Here's how the part is built. I have some questions about the finished solid (model axes, mm). A direction names the side the tool comes from. Coordinates: 2 decimals unless noted, no trailing zeros. Write each loop counter-clockwise with the first axis right and the second up, starting at its lowest first coordinate (ties: lowest second). Pieces come first, ordered by that corner, then holes. Notation, with made-up numbers: M 59.25,27 L 99.25,27 A30 cw 99.25,54 Z; hole C 7,75.25 d2. An arc over 180 degrees is marked long. Write each question's results on one line, items separated by ' | '. Start each with the question number.
from build123d import *

# Parameters (mm, degrees)
F1_DEPTH = 4.4958
F3_DEPTH = 3.175
F5_DEPTH = 3.175
F7_DEPTH = 2.54
F9_DEPTH = 24.004


with BuildPart() as f1:
    # F0 (on Top) → F1 (new body)
    with BuildSketch(Plane.XY):
        with BuildLine():
            Line((-10.254373, 5.965228), (-10.254373, -0.308572))
            Line((-10.254373, -0.308572), (-10.254373, -9.70656))
            Line((-10.254373, -9.70656), (-8.895473, -18.088572))
            Line((-8.895473, -18.088572), (9.214727, -18.088572))
            Line((9.214727, -18.088572), (10.573627, -9.70656))
            Line((10.573627, -9.70656), (10.573627, -0.308572))
            Line((10.573627, -0.308572), (10.573627, 5.965228))
            Line((10.573627, 5.965228), (10.573627, 6.803428))
            Line((10.573627, 6.803428), (8.071727, 6.803428))
            Line((8.071727, 6.803428), (8.071727, -1.197572))
            ThreePointArc((8.071727, -1.197572), (7.789027, -1.880072), (7.106527, -2.162772))
            ThreePointArc((7.106527, -2.162772), (6.424028, -1.880072), (6.141327, -1.197572))
            Line((6.141327, -1.197572), (6.141327, 6.803428))
            Line((6.141327, 6.803428), (-5.974473, 6.803428))
            Line((-5.974473, 6.803428), (-5.974473, -1.197572))
            ThreePointArc((-5.974473, -1.197572), (-6.257173, -1.880072), (-6.939673, -2.162772))
            ThreePointArc((-6.939673, -2.162772), (-7.622172, -1.880072), (-7.904873, -1.197572))
            Line((-7.904873, -1.197572), (-7.904873, 6.803428))
            Line((-7.904873, 6.803428), (-10.254373, 6.803428))
            Line((-10.254373, 6.803428), (-10.254373, 5.965228))
        make_face()
    extrude(amount=F1_DEPTH)

    # F2 (on face) → F3 (join)
    with BuildSketch(Plane.YZ.offset(10.573627)):
        with BuildLine():
            Line((4.555528, 2.2479), (4.555528, 4.2799))
            ThreePointArc((4.555528, 4.2799), (2.523528, 2.2479), (4.555528, 0.2159))
            Line((4.555528, 0.2159), (4.555528, 2.2479))
        make_face()
        with BuildLine():
            ThreePointArc((4.555528, 0.2159), (5.992369, 0.811059), (6.587528, 2.2479))
            ThreePointArc((6.587528, 2.2479), (5.992369, 3.684741), (4.555528, 4.2799))
            Line((4.555528, 4.2799), (4.555528, 2.2479))
            Line((4.555528, 2.2479), (4.555528, 0.2159))
        make_face()
    extrude(amount=F3_DEPTH)

    # F4 (on face) → F5 (join)
    with BuildSketch(Plane(origin=(-10.254373, 0, 0), x_dir=(0, -1, 0), z_dir=(-1, 0, 0))):
        with BuildLine():
            Line((-4.555528, 2.2479), (-4.555528, 4.2799))
            ThreePointArc((-4.555528, 4.2799), (-5.992369, 3.684741), (-6.587528, 2.2479))
            ThreePointArc((-6.587528, 2.2479), (-5.992369, 0.811059), (-4.555528, 0.2159))
            Line((-4.555528, 0.2159), (-4.555528, 2.2479))
        make_face()
        with BuildLine():
            ThreePointArc((-4.555528, 0.2159), (-3.118687, 0.811059), (-2.523528, 2.2479))
            ThreePointArc((-2.523528, 2.2479), (-3.118687, 3.684741), (-4.555528, 4.2799))
            Line((-4.555528, 4.2799), (-4.555528, 2.2479))
            Line((-4.555528, 2.2479), (-4.555528, 0.2159))
        make_face()
    extrude(amount=F5_DEPTH)

    # F6 (on face) → F7 (cut)
    with BuildSketch(Plane.XY.offset(4.4958)):
        with BuildLine():
            ThreePointArc((-5.974473, -1.197572), (-6.939673, -2.162772), (-7.904873, -1.197572))
            Line((-7.904873, -1.197572), (-7.904873, -9.70656))
            Line((-7.904873, -9.70656), (-6.545973, -18.088572))
            Line((-6.545973, -18.088572), (6.712827, -18.088572))
            Line((6.712827, -18.088572), (8.071727, -9.70656))
            Line((8.071727, -9.70656), (8.071727, -1.197572))
            ThreePointArc((8.071727, -1.197572), (7.106527, -2.162772), (6.141327, -1.197572))
            Line((6.141327, -1.197572), (6.141327, 6.803428))
            Line((6.141327, 6.803428), (-5.974473, 6.803428))
            Line((-5.974473, 6.803428), (-5.974473, -1.197572))
        make_face()
    extrude(amount=-F7_DEPTH, mode=Mode.SUBTRACT)

    # F8 (on face) → F9 (cut, through all)
    with BuildSketch(Plane.YZ.offset(10.573627)):
        Polygon((-18.088572, 4.4958), (-18.088572, 0), (-16.818572, 4.4958), align=None)
    extrude(amount=-F9_DEPTH, mode=Mode.SUBTRACT)


solid = f1.part
1) I want a section at D-D, the plane x = 8.5. Write out the boundary of the cut face in (y, z).
2) We'd pull the mould along X, two halves only. Please class faces 4 (the flat face through (10.574, -3, 2)), 5 (the flat face through (-7.905, 0, 3)), 6 (the flat face through (-9, 6.803, 2)): pulls with the +X half, pulls with the -X half, needs draft (parallel to the pull), parting line crosses it, or undercut.
3) I want a section at C-C, the plane y = -8.25. Write out the boundary of the cut face in (x, z).
4) I want a section at B-B, the plane z = 2.75. Write out the boundary of the cut face in (x, y), then the cut area to 3 significant figures.
5) For pin 1 Ø1.3 at (y, z) = (-3.5, 1) entering from -X; pin 2 Ø2 at (x, y) = (-3, -14.5) entering from +Z; pin 3 Ø2 at (y, z) = (-13.5, 2) entering from +X, each with a flat end and sliding along its axis, tell me the tip position at first contact or that it passes through.
6) For faces 1 (the flat face through (0, -5, 1.956)), 2 (the flat face through (9, 6.803, 2)), 3 (the flat face through (-5.974, 3, 1)), which set-ups out of +Z, -Z, +X, -X, +Y, -Y let a thin tool reach every point of the face, with its end or its side?
7) I want a section at A-A, the plane y = 1.5. Write out the boundary of the cut face in (x, z).
8) Please list where these lines run through material, in increasing order: line 1 (X direction, y = 2, z = 1.1); line 2 (X direction, y = 1.25, z = 3.25); line 3 (Z direction, x = -1.25, y = 0). Write a range as [from, to].
Output:
1) outline: M -18.09,0 L 6.8,0 L 6.8,4.5 L -16.82,4.5 Z
2) face 4: pulls with the +X half | face 5: undercut | face 6: needs draft
3) outline: M -10.25,0 L 10.57,0 L 10.57,4.5 L 8.07,4.5 L 8.07,1.96 L -7.9,1.96 L -7.9,4.5 L -10.25,4.5 Z
4) outline: M -13.43,2.59 L -10.25,2.59 L -10.25,-9.71 L -9.02,-17.31 L -6.67,-17.31 L -7.9,-9.71 L -7.9,6.8 L -10.25,6.8 L -10.25,6.52 L -13.43,6.52 Z; M 6.84,-17.31 L 9.34,-17.31 L 10.57,-9.71 L 10.57,2.59 L 13.75,2.59 L 13.75,6.52 L 10.57,6.52 L 10.57,6.8 L 8.07,6.8 L 8.07,-9.71 Z | area: 142 mm2
5) pin 1: stops at x = -10.25 | pin 2: stops at z = 1.96 | pin 3: stops at x = 10.12
6) face 1: +Z, +Y | face 2: +Z, -Z, +X, -X, +Y | face 3: +Z, -Z, +Y
7) outline: M -10.25,0 L -7.9,0 L -7.9,4.5 L -10.25,4.5 Z; M -5.97,0 L 6.14,0 L 6.14,1.96 L -5.97,1.96 Z; M 8.07,0 L 10.57,0 L 10.57,4.5 L 8.07,4.5 Z
8) line 1: x = [-10.25, -7.9], [-5.97, 6.14], [8.07, 10.57] | line 2: x = [-10.25, -7.9], [8.07, 10.57] | line 3: z = [0, 1.96]
